Geometry: final body of the model. Coordinates: model frame, mm. A direction names the side the tool comes from. Give positions to 0.01 mm unless a question says otherwise; leave off trailing zeros. Write each loop counter-clockwise with the first axis right and the second up, starting at its lowest first coordinate (ties: lowest second). Pieces come first, ordered by that corner, then holes. Notation, with made-up numbers: M -29,77.5 L 30,77.5 A19 cw 30,106.5 Z; hole C 6.25,-27 d2. An arc over 180 degrees is marked long. One line per question, with ' | ' between items.
Autodesk Inventor part; units mm, degrees
ref_plane "Work Plane3" through (0, 6.4, -20) normal (0, 1, 0) x (-1, 0, 0)
ref_plane "YZ Plane" through (0, 0, 0) normal (1, 0, 0) x (0, 1, 0)
ref_plane "XZ Plane" through (0, 0, 0) normal (0, 1, 0) x (-1, 0, 0)
sketch "Sketch1" plane through (0, 0, 0) normal (0, 1, 0) x (-1, 0, 0)
  line L0 (0, -40) -> (0, 0)
  line L1 (0, 0) -> (0, -18)
  circle A0 centre (0, -18) radius 1.55
  line L2 (0, -18) -> (0, -26.5)
  line L3 (0, -40) -> (0, -32)
  line L4 (0, -32) -> (1.5, -32)
  line L5 (1.5, -32) -> (1.5, -40)
  line L6 (0, 0) -> (6.4, 0)
  line L7 (6.4, 0) -> (6.4, -40)
  line L8 (6.4, -40) -> (1.5, -40)
  line L9 (6.4, -40) -> (7.9, -40)
  line L10 (7.9, -40) -> (7.9, 0)
  line L11 (7.9, 0) -> (6.4, 0)
  line L12 (6.4, 0) -> (4.9, 0)
  line L13 (4.9, 0) -> (4.9, -40)
  line L14 (4.9, -40) -> (6.4, -40)
  line L15 (0, 0) -> (3.15, 0)
  line L16 (3.15, 0) -> (3.15, -26.5)
  line L17 (3.15, -26.5) -> (0, -26.5)
  line L18 (7.9, 0) -> (7.9, -20)
  line L19 (7.9, -20) -> (6.4, -20)
  line L20 (6.4, -20) -> (4.9, -20)
  dimension "d3" = 18
  dimension "d4" = 3.1
  dimension "d5" = 8.5
  dimension "d6" = 8
  dimension "d7" = 1.5
  dimension "d22" = 6.4
  dimension "d27" = 1.5
  dimension "d28" = 1.5
  dimension "d35" = 3.15
  dimension "d45" = 20
revolve "Revolution3" add sketch "Sketch1" angle 360 about axis through (0, 0, 0) along (0, 0, -1) contours L0 L17 L16 L6 L13 L8 L5 L4 | L13 L20 L7 L8 | L6 L7 L20 L13
extrude "Extrusion8" cut sketch "Sketch1" along normal mid plane 15 contours A0 L0 | L0 A0
ref_plane "Work Plane3" through (0, 6.4, -20) normal (0, 1, 0) x (-1, 0, 0)
sketch "Sketch4" plane through (0, 6.4, -20) normal (0, 1, 0) x (-1, 0, 0)
  line L0 (0, 20) -> (0, 2)
  circle A0 centre (0, 2) radius 4
  dimension "d41" = 18
  dimension "d42" = 8
extrude "Extrusion9" cut sketch "Sketch4" against normal blind 3
extrude "Extrusion10" add sketch "Sketch1" along normal mid plane 3 contours L6 L7 L20 L13 | L11 L10 L19 L7
sketch "Sketch5" plane through (-7.9, 1.5, 0) normal (0, 0, 1) x (1, 0, 0)
  circle A0 centre (7.9, -1.5) radius 3.25
  circle A1 centre (7.9, -1.5) radius 1.5
  circle A2 centre (7.9, -1.5) radius 8.5
  dimension "d48" = 6.5
  dimension "d51" = 17
extrude "Extrusion11" cut sketch "Sketch5" against normal blind 26.5 contours A0 | A1
extrude "Extrusion12" add sketch "Sketch5" against normal blind 4.5 contours A2
properties part number "dc_to_omni_coupler"
(1) Set-up query: faces 4 (the face through (-7.9, 0, -12)), 5 (the face through (-2, 3.4, -18)), 6 (the face through (-7, 1.5, -12)). Return all of +Z, -Z, +X, -X, +Y, -Y with unobstructed straight access to the full face (end or side cutting, diameter ignored); none if empty.
Working result:
face 4: -Z, -X, +Y, -Y | face 5: +Y | face 6: -Z, -X, +Y
(2) Material intervals for L1, parallel to Z at x = 0, y = -5.45; L2, parallel to Y at x = 0.25, z = -25; L3, parallel to Z at x = 1.5, y = 7.5, sorted ascending. Write a range as [from, to].
Working result:
L1: z = [-40, -19.55], [-16.45, 0] | L2: y = [-6.4, -3.24], [3.24, 6.4] | L3: z = [-4.5, 0]
(3) Cut plane B-B, the plane z = -6.5. Return loops of the section in (x, y).
Working result:
outline: M -7.9,-1.5 L -6.22,-1.5 A6.4 ccw long -6.22,1.5 L -7.9,1.5 Z; hole C 0,0 d6.5
(4) Cut plane D-D, the plane y = 0. Return loops of the section in (x, z).
Working result:
outline: M -8.5,-4.5 L -7.9,-4.5 L -7.9,-20 L -6.4,-20 L -6.4,-40 L -1.5,-40 L -1.5,-32 L 1.5,-32 L 1.5,-40 L 6.4,-40 L 6.4,-4.5 L 8.5,-4.5 L 8.5,0 L 3.25,0 L 3.25,-26.5 L -3.25,-26.5 L -3.25,0 L -8.5,0 Z
(5) First-contact query: P1, Ø10, axis at x = 1.5, z = -16, coming from the -Y side; P2, Ø0.5, axis at x = -7, z = -11.5, coming from the +Y side; P3, Ø2.5, axis at x = 1, z = -19.5, coming from the +Y side. Flat tips, straight axial feed; report the tip coordinate or a pass-through.
Working result:
P1: stops at y = -6.4 | P2: stops at y = 1.5 | P3: stops at y = 3.4
(6) Cut plane C-C, the plane z = -17.5. Return loops of the section in (x, y), then the cut area to 3 significant figures.
Working result:
outline: M -7.9,-1.5 L -6.22,-1.5 A6.4 ccw -1.47,-6.23 L -1.47,-2.9 A3.25 cw -1.47,2.9 L -1.47,3.4 L -3.97,3.4 L -3.97,5.02 A6.4 ccw -6.22,1.5 L -7.9,1.5 Z; M 1.47,-6.23 A6.4 ccw 3.97,5.02 L 3.97,3.4 L 1.47,3.4 L 1.47,2.9 A3.25 cw 1.47,-2.9 Z | area: 69.7 mm^2
(7) Draft query along X for faces 1 (the face through (4, 0, 0)), 2 (the face through (1.387, -6.248, -22.498)), 3 (the face through (0, 0, -26.5)). Return one class per face: released by +X, released by -X, zero draft, split by the parting line, or undercut.
Working result:
face 1: zero draft | face 2: split by the parting line | face 3: undercut
(8) Cut plane A-A, the plane x = 0. Return loops of the section in (y, z).
Working result:
outline: M -8.5,-4.5 L -6.4,-4.5 L -6.4,-16.45 L -3.25,-16.45 L -3.25,0 L -8.5,0 Z; M -6.4,-40 L -1.5,-40 L -1.5,-32 L 1.5,-32 L 1.5,-40 L 6.4,-40 L 6.4,-22 L 3.4,-22 L 3.4,-19.55 L 3.25,-19.55 L 3.25,-26.5 L -3.25,-26.5 L -3.25,-19.55 L -6.4,-19.55 Z; M 3.25,-16.45 L 3.4,-16.45 L 3.4,-14 L 6.4,-14 L 6.4,-4.5 L 8.5,-4.5 L 8.5,0 L 3.25,0 Z
